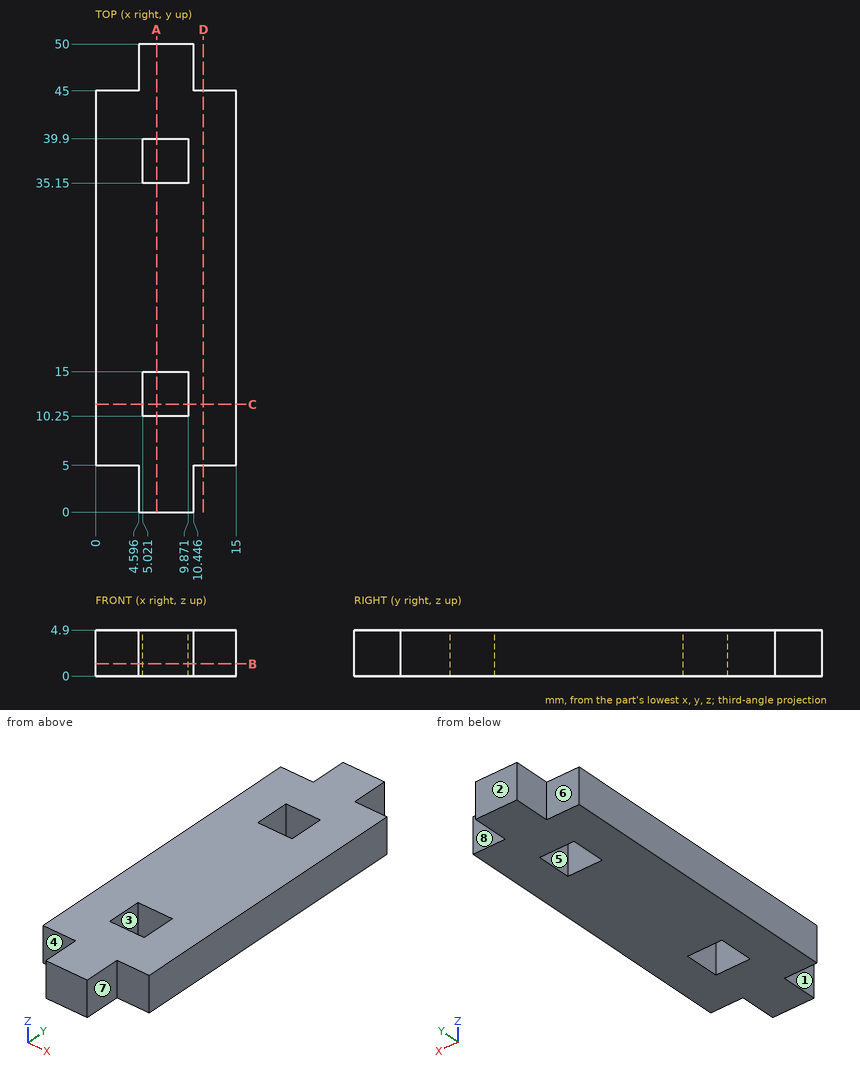
Geometry: see drawing. Coordinates: mm, zero at the bounding-box minimum. A direction names the side the tool comes from. Coordinates: 2 decimals unless noted, no trailing zeros. Loops run counter-clockwise (first coordinate to the right, second up) from the corner with the lowest first, then second, coordinate; pieces in that order, holes last. Notation, with made-up numbers: (31, 21.5) - (47, 21.5) arc R35 ccw to (47, 57.5) - close; hole circle Ø9 at (-36.75, -18). An arc over 180 degrees is marked (long way). Put each result on its own line as item: value. Start each with the question number.
Q1. Set-up query: the marked faces 4, 5, 6, 7 and 8. Return all of +Z, -Z, +X, -X, +Y, -Y with unobstructed straight access to the full face (end or side cutting, diameter ignored); none if empty.
Q2. Cut plane C-C, the plane y = 11.5. Return loops of the section in (x, z).
Q3. Cut plane D-D, the plane x = 11.5. Return loops of the section in (y, z), and give its area (3 significant figures).
Q4. Line query: line 1 (Y direction, x = 7.75, z = 2.4); line 2 (X direction, y = 37, z = 3.4); line 3 (X direction, y = 2, z = 3.35). Output: solid intervals per line, ascending.
Q5. Pin query (flat end, axial travel): pin 1 Ø1.5 at (x, y) = (12, 39.5) entering from -Z; pin 2 Ø1.4 at (x, z) = (13, 2) entering from +Y; pin 3 Ø1.4 at (x, z) = (14, 3.5) entering from -Y; pin 4 Ø1.5 at (y, z) = (3.5, 3.5) entering from -X. Return the tip coordinate at first contact, or that it passes through.
Q6. Cut plane B-B, the plane z = 1.3. Return loops of the section in (x, y).
Q7. Cut plane A-A, the plane x = 6.5. Return loops of the section in (y, z).
Q8. Pull-direction query (X, two-part tool) for the marked faces 1, 2 and 3; classes: released by +X, released by -X, zero draft, split by the parting line, or undercut.
Filled sheet:
1. face 4: +Z, -Z, -X, -Y
1. face 5: +Z, -Z
1. face 6: +Z, -Z, -X, +Y
1. face 7: +Z, -Z, +X, -Y
1. face 8: +Z, -Z, +X, +Y
2. outline: (0, 0) - (5.02, 0) - (5.02, 4.9) - (0, 4.9) - close; (9.87, 0) - (15, 0) - (15, 4.9) - (9.87, 4.9) - close
3. outline: (5, 0) - (45, 0) - (45, 4.9) - (5, 4.9) - close
3. area: 196 mm²
4. line 1: 0 to 10.25, 15 to 35.15, 39.9 to 50
4. line 2: 0 to 5.02, 9.87 to 15
4. line 3: 4.6 to 10.45
5. pin 1: z = 0
5. pin 2: y = 45
5. pin 3: y = 5
5. pin 4: x = 4.6
6. outline: (0, 5) - (4.6, 5) - (4.6, 0) - (10.45, 0) - (10.45, 5) - (15, 5) - (15, 45) - (10.45, 45) - (10.45, 50) - (4.6, 50) - (4.6, 45) - (0, 45) - close; hole (5.02, 10.25) - (9.87, 10.25) - (9.87, 15) - (5.02, 15) - close; hole (5.02, 35.15) - (9.87, 35.15) - (9.87, 39.9) - (5.02, 39.9) - close
7. outline: (0, 0) - (10.25, 0) - (10.25, 4.9) - (0, 4.9) - close; (15, 0) - (35.15, 0) - (35.15, 4.9) - (15, 4.9) - close; (39.9, 0) - (50, 0) - (50, 4.9) - (39.9, 4.9) - close
8. face 1: released by -X
8. face 2: zero draft
8. face 3: undercut
